```python
from build123d import *

# Parameters (mm, degrees)
F0_W     = 216
F0_H     = 50
F1_DEPTH = 2
F3_DEPTH = 2
F4_W     = 32
F4_H     = 82.0060973343
F5_DEPTH = 2
F7_DEPTH = 2
F8_W     = 32
F8_H     = 82.0060973343
F9_DEPTH = 2
F10_R    = 5


# Not quite as in the source:
# - a feature names something its author has since deleted; it is built from what else it names


with BuildPart() as f1:
    # F0 (on Front) → F1 (new body)
    with BuildSketch(Plane.XZ):
        Rectangle(F0_W, F0_H)
        with BuildLine():
            ThreePointArc((-27.5, -10.5), (-24.6715728753, -11.6715728753), (-23.5, -14.5))
            ThreePointArc((-23.5, -14.5), (-24.6715728753, -17.3284271247), (-27.5, -18.5))
            Line((-27.5, -18.5), (-52.5, -18.5))
            ThreePointArc((-52.5, -18.5), (-56.5, -14.5), (-52.5, -10.5))
            Line((-52.5, -10.5), (-27.5, -10.5))
        make_face(mode=Mode.SUBTRACT)
        with BuildLine():
            ThreePointArc((27.5, -18.5), (23.5, -14.5), (27.5, -10.5))
            Line((27.5, -10.5), (52.5, -10.5))
            ThreePointArc((52.5, -10.5), (55.3284271247, -11.6715728753), (56.5, -14.5))
            ThreePointArc((56.5, -14.5), (55.3284271247, -17.3284271247), (52.5, -18.5))
            Line((52.5, -18.5), (27.5, -18.5))
        make_face(mode=Mode.SUBTRACT)
        with BuildLine():
            ThreePointArc((-52.5, 10.5), (-56.5, 14.5), (-52.5, 18.5))
            Line((-52.5, 18.5), (-27.5, 18.5))
            ThreePointArc((-27.5, 18.5), (-24.6715728753, 17.3284271247), (-23.5, 14.5))
            ThreePointArc((-23.5, 14.5), (-24.6715728753, 11.6715728753), (-27.5, 10.5))
            Line((-27.5, 10.5), (-52.5, 10.5))
        make_face(mode=Mode.SUBTRACT)
        with BuildLine():
            ThreePointArc((27.5, 10.5), (23.5, 14.5), (27.5, 18.5))
            Line((27.5, 18.5), (52.5, 18.5))
            ThreePointArc((52.5, 18.5), (55.3284271247, 17.3284271247), (56.5, 14.5))
            ThreePointArc((56.5, 14.5), (55.3284271247, 11.6715728753), (52.5, 10.5))
            Line((52.5, 10.5), (27.5, 10.5))
        make_face(mode=Mode.SUBTRACT)
    extrude(amount=-F1_DEPTH)

    # F2 (on face) → F3 (join)
    with BuildSketch(Plane(origin=(-108, 0, 0), x_dir=(0, -1, 0), z_dir=(-1, 0, 0))):
        Polygon((0, 25), (0, -25), (115, -25), (50, 25), align=None)
    extrude(amount=-F3_DEPTH)

    # F4 (on face) → F5 (join)
    with BuildSketch(Plane(origin=(0, -30.6691449814, 39.8698884758), x_dir=(1, 0, 0), z_dir=(0, -0.6097107608, 0.7926239891))):
        with Locations((-122, -65.3914791011)):
            Rectangle(F4_W, F4_H)
        with BuildLine():
            ThreePointArc((-119.5, -96.8914791011), (-117.0251262658, -97.916605367), (-116, -100.3914791011))
            ThreePointArc((-116, -100.3914791011), (-117.0251262658, -102.8663528353), (-119.5, -103.8914791011))
            Line((-119.5, -103.8914791011), (-131.5, -103.8914791011))
            ThreePointArc((-131.5, -103.8914791011), (-135, -100.3914791011), (-131.5, -96.8914791011))
            Line((-131.5, -96.8914791011), (-119.5, -96.8914791011))
        make_face(mode=Mode.SUBTRACT)
        with BuildLine():
            ThreePointArc((-131.5, -33.8914791011), (-135, -30.3914791011), (-131.5, -26.8914791011))
            Line((-131.5, -26.8914791011), (-119.5, -26.8914791011))
            ThreePointArc((-119.5, -26.8914791011), (-117.0251262658, -27.916605367), (-116, -30.3914791011))
            ThreePointArc((-116, -30.3914791011), (-117.0251262658, -32.8663528353), (-119.5, -33.8914791011))
            Line((-119.5, -33.8914791011), (-131.5, -33.8914791011))
        make_face(mode=Mode.SUBTRACT)
    extrude(amount=F5_DEPTH)

    # F6 (on face) → F7 (join)
    with BuildSketch(Plane.YZ.offset(108)):
        Polygon((0, -25), (0, 25), (-50, 25), (-115, -25), align=None)
    extrude(amount=-F7_DEPTH)

    # F8 (on face) → F9 (join)
    with BuildSketch(Plane(origin=(0, -30.6691449814, 39.8698884758), x_dir=(1, 0, 0), z_dir=(0, -0.6097107608, 0.7926239891))):
        with Locations((122, -65.3914791011)):
            Rectangle(F8_W, F8_H)
        with BuildLine():
            ThreePointArc((131.5, -96.8914791011), (133.9748737342, -97.916605367), (135, -100.3914791011))
            ThreePointArc((135, -100.3914791011), (133.9748737342, -102.8663528353), (131.5, -103.8914791011))
            Line((131.5, -103.8914791011), (119.5, -103.8914791011))
            ThreePointArc((119.5, -103.8914791011), (116, -100.3914791011), (119.5, -96.8914791011))
            Line((119.5, -96.8914791011), (131.5, -96.8914791011))
        make_face(mode=Mode.SUBTRACT)
        with BuildLine():
            ThreePointArc((119.5, -33.8914791011), (116, -30.3914791011), (119.5, -26.8914791011))
            Line((119.5, -26.8914791011), (131.5, -26.8914791011))
            ThreePointArc((131.5, -26.8914791011), (133.9748737342, -27.916605367), (135, -30.3914791011))
            ThreePointArc((135, -30.3914791011), (133.9748737342, -32.8663528353), (131.5, -33.8914791011))
            Line((131.5, -33.8914791011), (119.5, -33.8914791011))
        make_face(mode=Mode.SUBTRACT)
    extrude(amount=F9_DEPTH)

    # F10
    f10_edges = [f1.edges().sort_by_distance(p)[0] for p in [
        (-106, -83.719422, 1.585248),
        (-108, -82.5, 0),
        (-108, 2, 0),
        (-106, 0, 0),
        (106, 0, 0),
        (108, 2, 0),
        (108, -82.5, 0),
        (-138, -115.609711, -24.207376),
        (-138, -50.609711, 25.792624),
        (106, -83.719422, 1.585248),
        (138, -50.609711, 25.792624),
        (138, -115.609711, -24.207376),
    ]]
    fillet(f10_edges, radius=F10_R)


solid = f1.part
```
For this review, take the finished solid that the model builds, in its own axes (mm). A direction names the side the tool comes from. Coordinates: 2 decimals unless noted, no trailing zeros. Write each loop counter-clockwise with the first axis right and the second up, starting at its lowest first coordinate (ties: lowest second). Pieces come first, ordered by that corner, then holes. Notation, with made-up numbers: (39.5, 5.5) - (80.5, 5.5) arc R25 cw to (80.5, 39.5) - close; hole circle Ø7 at (-31.75, 63.5). An arc over 180 degrees is marked (long way). Answer in a Markdown table with one row per item. Add a question column.
Q1. For P1, Ø25, axis at y = -62, z = 11, coming from the +X side; P2, Ø10, axis at y = -40.5, z = -2.5, coming from the -X side; P3, Ø3, axis at x = -92, z = 18.5, coming from the -Y side; P4, Ø2, axis at x = -37.5, y = 1.5, coming from the +Z side, all flat-tipped, find the tip position at first contact; note any pin that passes through.
Q2. For probe 1 along X at (y, z) = (-22, 10); probe 2 along Y at (x, z) = (89, -18.5); probe 3 along Y at (x, z) = (105.5, 9), list the stretches that pass through material, from the lowest coordinate up.
Q3. We need section A-A, the plane y = -28. State the section outline as (x, z) points, and give its area (3 significant figures).
Q4. We need section B-B, the plane x = -11. State the section outline as (y, z) points, and give its area (3 significant figures).
Q5. Draft analysis for pull direction X (two halves, no side actions). For faces 4 (the cylindrical face through (-135, -110.9, -20.6)), 5 (the cylindrical face through (107.4, -80.8, 1.9)), 6 (the flat face through (-124.69, -83.26, 1.94)), 7 (the flat face through (138, -84, 0)), state which applies: +X half, -X half, draft (parallel to the pull), parting line (faces both ways), or undercut.
Q6. Tool access review of faces 1 (the cylindrical face through (116, -55.4, 22.1)), 2 (the flat face through (-8, 1, 25)), 3 (the flat face through (125.325, -82.045, 0.35)): name each direction out of +Z, -Z, +X, -X, +Y, -Y from which nothing blocks a thin tool from reaching the whole face with its end or side.
Answer list:
| question | item | result |
|---|---|---|
| 1 | P1 | stops at x = 138 |
| 1 | P2 | stops at x = -108 |
| 1 | P3 | stops at y = 0 |
| 1 | P4 | stops at z = 25 |
| 2 | probe 1 | x = -108 to -106, 106 to 108 |
| 2 | probe 2 | y = 0 to 2 |
| 2 | probe 3 | y = -2.82 to 1.33 |
| 3 | outline | (-108, -25) - (-106, -25) - (-106, 25) - (-108, 25) - close; (106, -25) - (108, -25) - (108, 25) - (106, 25) - close |
| 3 | area | 200 mm2 |
| 4 | outline | (0, -25) - (2, -25) - (2, 25) - (0, 25) - close |
| 4 | area | 100 mm2 |
| 5 | face 4 | undercut |
| 5 | face 5 | undercut |
| 5 | face 6 | draft |
| 5 | face 7 | +X half |
| 6 | face 1 | none |
| 6 | face 2 | +Z, +X, -X, +Y |
| 6 | face 3 | -Z, +X, +Y |
